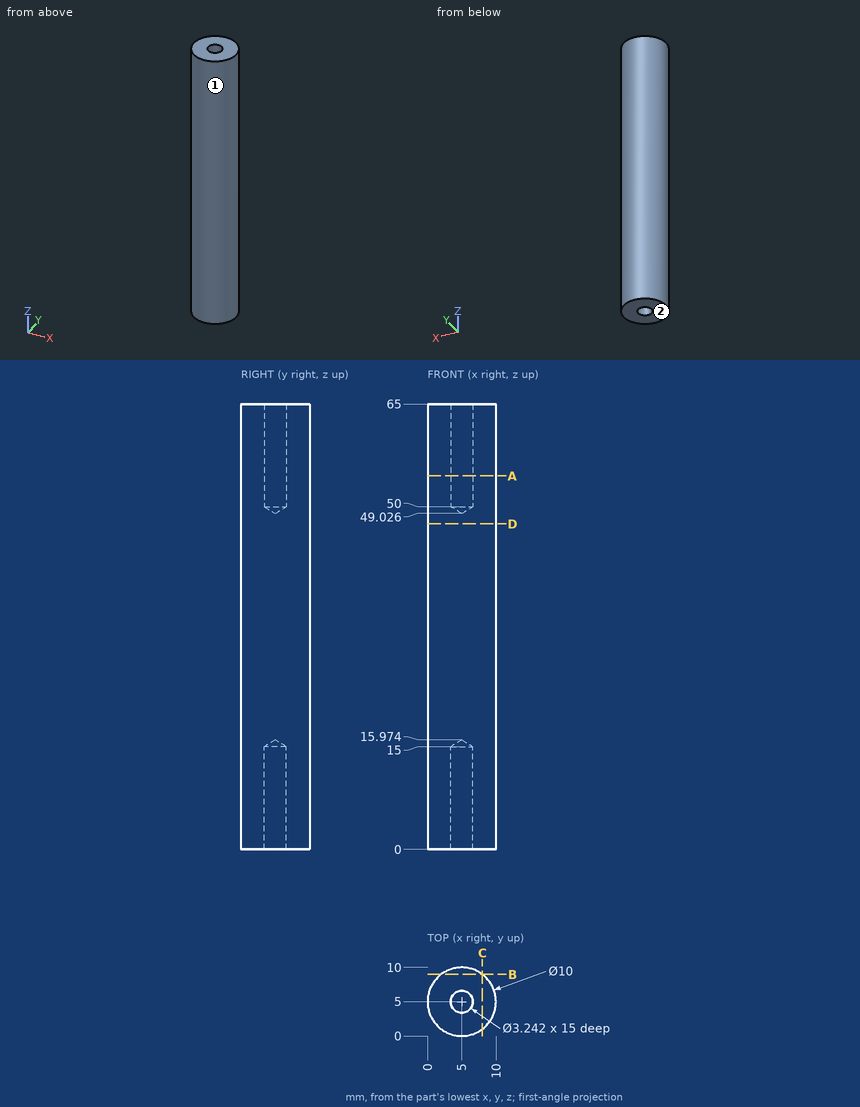
Could you check a few things on this drawing? It's one solid part, dimensions in mm from its lowest x, y, z. Coordinates: 2 decimals unless noted, no trailing zeros. Loops run counter-clockwise (first coordinate to the right, second up) from the corner with the lowest first, then second, coordinate; pieces in that order, holes last. Notation, with made-up numbers: (18, 46.5) - (42, 46.5) arc R19 ccw to (42, 71.5) - close; hole circle Ø11 at (75, 8). An arc over 180 degrees is marked (long way). Answer as a JSON object with one key per item and string values. Group by question number.
Item 1: For pin 1 (1.9 mm diameter, centred on x = 5, y = 5, fed in from -Z); pin 2 (1.5 mm diameter, centred on x = 3.5, z = 14.5, fed in from -Y); pin 3 (1.5 mm diameter, centred on y = 2.5, z = 56.5, fed in from -X), each with a flat end and sliding along its axis, tell me the tip position at first contact or that it passes through.
Item 2: If we section it at D-D (z = 47.5): List the corners of the cut face in (x, y) for me, plus the area to 3 significant figures.
Item 3: If I drill on L1, parallel to Y at x = 5, z = 58.5; L2, parallel to X at y = 6, z = 59; L3, parallel to X at y = 3.75, z = 7, over which ranges is the centre line in solid material (lowest first)? Write a range as from..to.
Item 4: If we mould it in two halves opening along X, with no side actions, what happens to the marked faces 1 and 2? For each: released by +X, released by -X, zero draft, split by the parting line, or undercut.
Item 5: If we section it at B-B (y = 9): List the corners of the cut face in (x, z) for me, plus the area to 3 significant figures.
Item 6: If we section it at C-C (x = 8): List the corners of the cut face in (y, z) for me, plus the area to 3 significant figures.
Item 7: If we section it at A-A (z = 54.5): List the corners of the cut face in (x, y) for me.
Returned:
{
 "1": {"pin 1": "stops at z = 15.4", "pin 2": "stops at y = 0.06", "pin 3": "stops at x = 0.32"},
 "2": {"outline": "circle Ø10 at (5, 5)", "area": "78.5 mm²"},
 "3": {"L1": "y = 0..3.38, 6.62..10", "L2": "x = 0.1..3.72, 6.28..9.9", "L3": "x = 0.16..3.97, 6.03..9.84"},
 "4": {"face 1": "split by the parting line", "face 2": "zero draft"},
 "5": {"outline": "(2, 0) - (8, 0) - (8, 65) - (2, 65) - close", "area": "390 mm²"},
 "6": {"outline": "(1, 0) - (9, 0) - (9, 65) - (1, 65) - close", "area": "520 mm²"},
 "7": {"outline": "circle Ø10 at (5, 5); hole circle Ø3.24 at (5, 5)"}
}
